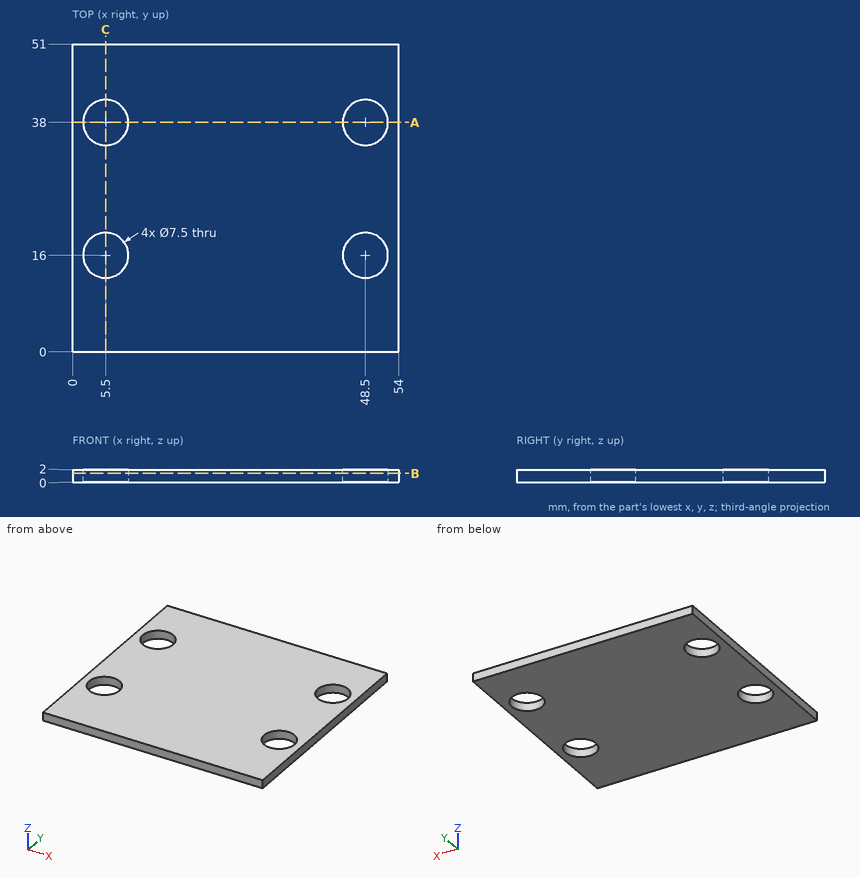
Input: dimensioned drawing with shaded views. Units: mm. Origin: part minimum x, y, z. Coordinates: 2 decimals unless noted, no trailing zeros. Write each loop counter-clockwise with the first axis right and the second up, starting at its lowest first coordinate (ties: lowest second). Pieces come first, ordered by that corner, then holes. Notation, with made-up numbers: M -35.5,-26.5 L 19.5,-26.5 A15 ccw 19.5,2.5 Z; hole C 44.5,6.5 d9. An arc over 180 degrees is marked long. Answer as a JSON object with one key per item and string values. Group by question number.
(1) Section C-C on x = 5.5. Output: boundary loops of the cut face in (y, z).
(2) Ray query, line 1 along Y through (x, z) = (48.5, 0.65); line 2 along Y through (x, z) = (51, 0.75); line 3 along X through (y, z) = (13.5, 1.35). Return the intervals inside material, ascending. Write a range as [from, to].
(3) Section B-B on z = 1.45. Output: boundary loops of the cut face in (x, y).
(4) Section A-A on y = 38. Output: boundary loops of the cut face in (x, z).
Result set:
{
 "1": {"outline": "M 0,0 L 12.25,0 L 12.25,2 L 0,2 Z; M 19.75,0 L 34.25,0 L 34.25,2 L 19.75,2 Z; M 41.75,0 L 51,0 L 51,2 L 41.75,2 Z"},
 "2": {"line 1": "y = [0, 12.25], [19.75, 34.25], [41.75, 51]", "line 2": "y = [0, 13.2], [18.8, 35.2], [40.8, 51]", "line 3": "x = [0, 2.7], [8.3, 45.7], [51.3, 54]"},
 "3": {"outline": "M 0,0 L 54,0 L 54,51 L 0,51 Z; hole C 5.5,16 d7.5; hole C 5.5,38 d7.5; hole C 48.5,16 d7.5; hole C 48.5,38 d7.5"},
 "4": {"outline": "M 0,0 L 1.75,0 L 1.75,2 L 0,2 Z; M 9.25,0 L 44.75,0 L 44.75,2 L 9.25,2 Z; M 52.25,0 L 54,0 L 54,2 L 52.25,2 Z"}
}
